Could you check a few things on this drawing? It's one solid part, dimensions in mm from its lowest x, y, z. A direction names the side the tool comes from. Coordinates: 2 decimals unless noted, no trailing zeros. Write each loop counter-clockwise with the first axis right and the second up, starting at its lowest first coordinate (ties: lowest second). Pieces come first, ordered by that corner, then holes.
Item 1: I'm going to push flat-ended pins straight in: P1, Ø3, axis at x = 4.5, z = 37.5, coming from the +Y side; P2, Ø1.8, axis at x = 8.5, y = 7.5, coming from the -Z side; P3, Ø1.5, axis at x = 6.5, y = 2, coming from the -Z side. Where does each tip first touch, or does it pass through?
Item 2: I want a section at D-D (z = 20.5). Please give me the cut outline in (x, y), and give its area (3 significant figures).
Item 3: Please list where these lines run through material, in increasing order: line 1 (Y direction, x = 8, z = 5); line 2 (Z direction, x = 4.5, y = 3.25); line 3 (Y direction, x = 9.5, z = 9.5).
Item 4: If we mould it in two halves opening along Y, with no side actions, what happens to the marked faces 3, 4 and 5? For each: pulls with the +Y half, pulls with the -Y half, needs draft (parallel to the pull), parting line crosses it, or undercut.
Item 5: I want a section at A-A (x = 8). Please give me the cut outline in (y, z).
Item 6: For the marked faces 1 and 2, which set-ups out of +Z, -Z, +X, -X, +Y, -Y let a thin tool reach every point of the face, with its end or its side?
Item 7: I want a section at C-C (z = 9). Please give me the cut outline in (x, y).
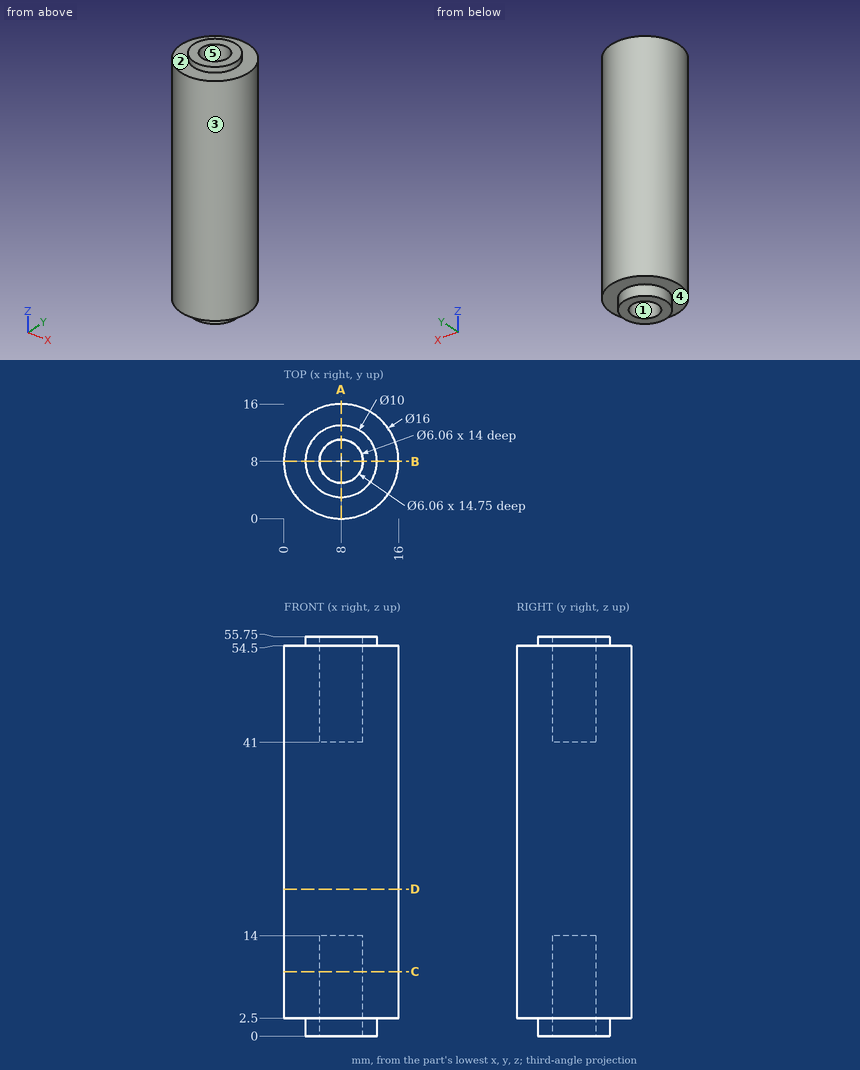
Answer:
1. P1: stops at y = 15.75
1. P2: stops at z = 14
1. P3: stops at z = 2.5
2. outline: circle Ø16 at (8, 8)
2. area: 201 mm2
3. line 1: y = 0 to 4.97, 11.03 to 16
3. line 2: z = 2.5 to 54.5
3. line 3: y = 0.14 to 5.37, 10.63 to 15.86
4. face 3: parting line crosses it
4. face 4: needs draft
4. face 5: undercut
5. outline: (0, 2.5) - (3, 2.5) - (3, 0) - (4.97, 0) - (4.97, 14) - (11.03, 14) - (11.03, 0) - (13, 0) - (13, 2.5) - (16, 2.5) - (16, 54.5) - (13, 54.5) - (13, 55.75) - (11.03, 55.75) - (11.03, 41) - (4.97, 41) - (4.97, 55.75) - (3, 55.75) - (3, 54.5) - (0, 54.5) - close
6. face 1: -Z
6. face 2: +Z
7. outline: circle Ø16 at (8, 8); hole circle Ø6.06 at (8, 8)
